Check sheet for the modelled part. Datum: model origin and axes. Units: mm. Face numbers are marked on the shaded views. Give positions to 0.01 mm unless a question says otherwise; leave off trailing zeros. Write each loop counter-clockwise with the first axis right and the second up, starting at its lowest first coordinate (ties: lowest second). Pieces come first, ordered by that corner, then holes.
from build123d import *

# Parameters (mm, degrees)
F0_W     = 76.2
F0_H     = 152.4
F1_DEPTH = 25.4
F2_W     = 65.024
F2_H     = 12.7
F3_DEPTH = 136.525
F4_R     = 5.08
F5_W     = 58.42
F5_H     = 104.14
F6_DEPTH = 7.62


with BuildPart() as f1:
    # F0 (on Front) → F1 (new body)
    with BuildSketch(Plane.XZ):
        with Locations((2.724684, -0.652284)):
            Rectangle(F0_W, F0_H)
    extrude(amount=F1_DEPTH)

    # F2 (on face) → F3 (cut)
    with BuildSketch(Plane.XY.offset(75.547716)):
        with Locations((2.623657, -11.599738)):
            Rectangle(F2_W, F2_H)
    extrude(amount=-F3_DEPTH, mode=Mode.SUBTRACT)

    # F4
    f4_edges = [f1.edges().sort_by_distance(p)[0] for p in [
        (40.824684, -25.4, -0.652284),
        (40.824684, 0, -0.652284),
        (-35.375316, 0, -0.652284),
        (-35.375316, -25.4, -0.652284),
        (2.724684, -25.4, -76.852284),
        (-35.375316, -12.7, -76.852284),
        (40.824684, -12.7, -76.852284),
        (2.724684, 0, -76.852284),
        (2.724684, -25.4, 75.547716),
        (-35.375316, -12.7, 75.547716),
        (40.824684, -12.7, 75.547716),
        (2.724684, 0, 75.547716),
    ]]
    fillet(f4_edges, radius=F4_R)

    # F5 (on face) → F6 (cut)
    with BuildSketch(Plane.XZ.offset(25.4)):
        with Locations((2.397154, 0.125338)):
            Rectangle(F5_W, F5_H)
    extrude(amount=-F6_DEPTH, mode=Mode.SUBTRACT)


solid = f1.part
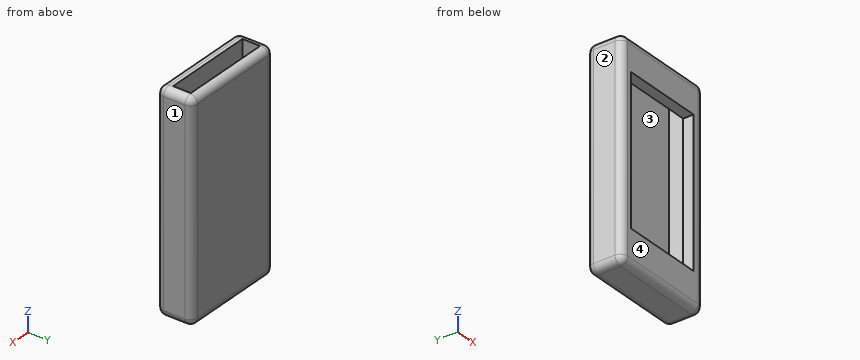
1) Gauge pin test, flat ends, axial feed: pin 1 (1 mm diameter, centred on x = -27.5, y = -3, fed in from -Z); pin 2 (6 mm diameter, centred on x = 5, z = -20.5, fed in from -Y); pin 3 (6.5 mm diameter, centred on x = -8, y = -9, fed in from +Z). Record the tip position at first contact, or that the pin passes through.
2) Scan lines: L1, parallel to X at y = -18, z = 32.5; L2, parallel to X at y = -6.5, z = 43.5; L3, parallel to Z at x = 11, y = -6.5. Record each from-to range of solid material in increasing order.
3) Sectioned sample at A-A on x = -20. Record the boundary of the cut face in (y, z).
4) Sectioned sample at B-B on z = -49. Record the boundary of the cut face in (x, y), then the cut area to 3 significant figures.
5) Draft check along X on the marked faces 1, 2, 3 and 4. Enter one of: +X half, -X half, draft (parallel to the pull), parting line (faces both ways), or undercut.
6) Sectioned sample at C-C on y = -15. Record the boundary of the cut face in (x, z), then the cut area to 3 significant figures.
Answers below:
1. pin 1: stops at z = -76.6
1. pin 2: stops at y = -5.25
1. pin 3: stops at z = -60.98
2. L1: x = -35.38 to -26.81, 31.61 to 40.82
2. L2: x = -35.38 to -29.89, 35.14 to 40.82
2. L3: z = -76.85 to -60.98
3. outline: (-25.4, -71.77) arc R5.08 ccw to (-20.32, -76.85) - (-5.08, -76.85) arc R5.08 ccw to (0, -71.77) - (0, 70.47) arc R5.08 ccw to (-5.08, 75.55) - (-5.25, 75.55) - (-5.25, -60.98) - (-17.95, -60.98) - (-17.95, -51.94) - (-25.4, -51.94) - close; (-25.4, 52.2) - (-17.95, 52.2) - (-17.95, 75.55) - (-20.32, 75.55) arc R5.08 ccw to (-25.4, 70.47) - close
4. outline: (-35.38, -20.32) arc R5.08 ccw to (-30.3, -25.4) - (-26.81, -25.4) - (-26.81, -17.95) - (-29.89, -17.95) - (-29.89, -5.25) - (35.14, -5.25) - (35.14, -17.95) - (31.61, -17.95) - (31.61, -25.4) - (35.74, -25.4) arc R5.08 ccw to (40.82, -20.32) - (40.82, -5.08) arc R5.08 ccw to (35.74, 0) - (-30.3, 0) arc R5.08 ccw to (-35.38, -5.08) - close
4. area: 652 mm2
5. face 1: +X half
5. face 2: -X half
5. face 3: undercut
5. face 4: draft
6. outline: (-35.38, -71.77) arc R5.08 ccw to (-30.3, -76.85) - (35.74, -76.85) arc R5.08 ccw to (40.82, -71.77) - (40.82, 70.47) arc R5.08 ccw to (35.74, 75.55) - (35.14, 75.55) - (35.14, -60.98) - (-29.89, -60.98) - (-29.89, 75.55) - (-30.3, 75.55) arc R5.08 ccw to (-35.38, 70.47) - close
6. area: 2,710 mm2
